```python
from build123d import *

# Parameters (mm, degrees)
SKETCH1_W                = 161
SKETCH1_H                = 100
BOSS_EXTRUDE1_DEPTH      = 12.75
BOSS_EXTRUDE1_DEPTH_BACK = 12.75
SKETCH2_R                = 6.63
SKETCH2_R_2              = 3.525
SKETCH2_R_3              = 1.975
CUT_EXTRUDE1_DEPTH       = 101
FILLET1_R                = 1
FILLET2_R                = 1
FILLET3_R                = 1
FILLET4_R                = 1
SKETCH3_R                = 2.5
BOSS_EXTRUDE2_DEPTH      = 10
SKETCH4_R                = 1.45
CUT_EXTRUDE2_DEPTH       = 5
SKETCH5_W                = 6
SKETCH5_H                = 13
CUT_EXTRUDE3_DEPTH       = 19.25
SKETCH6_R                = 10.25
CUT_EXTRUDE4_DEPTH       = 43.477415469
SKETCH8_R                = 1.5
CUT_EXTRUDE5_DEPTH       = 36.5
SKETCH11_R               = 3
BOSS_EXTRUDE4_DEPTH      = 5
SKETCH12_R               = 1.5
CUT_EXTRUDE7_DEPTH       = 5
SKETCH13_W               = 18.25
SKETCH13_H               = 6
BOSS_EXTRUDE5_DEPTH      = 100
SKETCH14_W               = 4
SKETCH14_H               = 2
BOSS_EXTRUDE6_DEPTH      = 25
BOSS_EXTRUDE6_DEPTH_BACK = 125


with BuildPart() as part:
    # Sketch1 → Boss-Extrude1 (new body, two sides)
    with BuildSketch(Plane(origin=(0, 0, 0), x_dir=(1, 0, 0), z_dir=(0, 1, 0))) as boss_extrude1_sk:
        Rectangle(SKETCH1_W, SKETCH1_H)
    extrude(amount=BOSS_EXTRUDE1_DEPTH)
    extrude(boss_extrude1_sk.sketch, amount=-BOSS_EXTRUDE1_DEPTH_BACK)

    # Sketch2 → Cut-Extrude1 (cut, through all)
    with BuildSketch(Plane.XY.offset(50)):
        with Locations((-67.75, 0)):
            Circle(SKETCH2_R)
        with Locations((67.75, 0)):
            Circle(SKETCH2_R_2)
        with Locations((-75.45, 8.2)):
            Circle(SKETCH2_R_3)
        with Locations((-75.45, -8.2)):
            Circle(SKETCH2_R_3)
        with Locations((-60.05, -8.2)):
            Circle(SKETCH2_R_3)
        with Locations((-60.05, 8.2)):
            Circle(SKETCH2_R_3)
    extrude(amount=-CUT_EXTRUDE1_DEPTH, mode=Mode.SUBTRACT)

    # Fillet1
    fillet1_edges = [part.edges().sort_by_distance(p)[0] for p in [
        (-74.38, 0, -50),
    ]]
    fillet(fillet1_edges, radius=FILLET1_R)

    # Fillet2
    fillet2_edges = [part.edges().sort_by_distance(p)[0] for p in [
        (-74.38, 0, 50),
    ]]
    fillet(fillet2_edges, radius=FILLET2_R)

    # Fillet3
    fillet3_edges = [part.edges().sort_by_distance(p)[0] for p in [
        (64.225, 0, 50),
    ]]
    fillet(fillet3_edges, radius=FILLET3_R)

    # Fillet4
    fillet4_edges = [part.edges().sort_by_distance(p)[0] for p in [
        (64.225, 0, -50),
    ]]
    fillet(fillet4_edges, radius=FILLET4_R)

    # Sketch3 → Boss-Extrude2 (add)
    with BuildSketch(Plane(origin=(0, 12.75, 0), x_dir=(1, 0, 0), z_dir=(0, 1, 0))):
        with Locations((-16.76, 42.46)):
            Circle(SKETCH3_R)
        with Locations((58.37, 42.46)):
            Circle(SKETCH3_R)
        with Locations((-17, -5.8)):
            Circle(SKETCH3_R)
        with Locations((34.7, -0.9)):
            Circle(SKETCH3_R)
        with Locations((65.72, -5.8)):
            Circle(SKETCH3_R)
    extrude(amount=BOSS_EXTRUDE2_DEPTH)

    # Sketch4 → Cut-Extrude2 (cut)
    with BuildSketch(Plane(origin=(0, 22.75, 0), x_dir=(1, 0, 0), z_dir=(0, 1, 0))):
        with Locations((-16.76, 42.46)):
            Circle(SKETCH4_R)
        with Locations((-17, -5.8)):
            Circle(SKETCH4_R)
        with Locations((34.7, -0.9)):
            Circle(SKETCH4_R)
        with Locations((65.72, -5.8)):
            Circle(SKETCH4_R)
        with Locations((58.37, 42.46)):
            Circle(SKETCH4_R)
    extrude(amount=-CUT_EXTRUDE2_DEPTH, mode=Mode.SUBTRACT)

    # Sketch5 → Cut-Extrude3 (cut)
    with BuildSketch(Plane(origin=(80.5, 0, 0), x_dir=(0, 0, -1), z_dir=(1, 0, 0))):
        with Locations((-30, 0)):
            Rectangle(SKETCH5_W, SKETCH5_H)
        with Locations((-10, 0)):
            Rectangle(SKETCH5_W, SKETCH5_H)
        with Locations((10, 0)):
            Rectangle(SKETCH5_W, SKETCH5_H)
        with Locations((30, 0)):
            Rectangle(SKETCH5_W, SKETCH5_H)
    extrude(amount=-CUT_EXTRUDE3_DEPTH, mode=Mode.SUBTRACT)

    # Sketch6 → Cut-Extrude4 (cut, through all)
    with BuildSketch(Plane(origin=(0, 20.916044041, 3.688062894), x_dir=(1, 0, 0), z_dir=(0, 0.984807753, 0.173648178))):
        with Locations((0, -21.249093385)):
            Circle(SKETCH6_R)
    extrude(amount=-CUT_EXTRUDE4_DEPTH, mode=Mode.SUBTRACT)

    # Sketch8 → Cut-Extrude5 (cut, through all)
    with BuildSketch(Plane.XZ.offset(12.75)):
        with Locations((28.5, 2.93086019)):
            Circle(SKETCH8_R)
        with Locations((28.5, 45.38111272)):
            Circle(SKETCH8_R)
        with Locations((-28.5, 2.93086019)):
            Circle(SKETCH8_R)
        with Locations((-28.5, 45.38111272)):
            Circle(SKETCH8_R)
    extrude(amount=-CUT_EXTRUDE5_DEPTH, mode=Mode.SUBTRACT)

    # Sketch11 → Boss-Extrude4 (add)
    with BuildSketch(Plane(origin=(0, 12.75, 0), x_dir=(1, 0, 0), z_dir=(0, 1, 0))):
        with Locations((-38, -6.5)):
            Circle(SKETCH11_R)
        with Locations((-38, -44)):
            Circle(SKETCH11_R)
        with Locations((-75.5, -6.5)):
            Circle(SKETCH11_R)
        with Locations((-75.5, -44)):
            Circle(SKETCH11_R)
    extrude(amount=BOSS_EXTRUDE4_DEPTH)

    # Sketch12 → Cut-Extrude7 (cut)
    with BuildSketch(Plane(origin=(0, 17.75, 0), x_dir=(1, 0, 0), z_dir=(0, 1, 0))):
        with Locations((-75.5, -44)):
            Circle(SKETCH12_R)
        with Locations((-75.5, -6.5)):
            Circle(SKETCH12_R)
        with Locations((-38, -6.5)):
            Circle(SKETCH12_R)
        with Locations((-38, -44)):
            Circle(SKETCH12_R)
    extrude(amount=-CUT_EXTRUDE7_DEPTH, mode=Mode.SUBTRACT)

    # Sketch13 → Boss-Extrude5 (add)
    with BuildSketch(Plane.XY.offset(50)):
        with Locations((89.625, 9.75)):
            Rectangle(SKETCH13_W, SKETCH13_H)
    extrude(amount=-BOSS_EXTRUDE5_DEPTH)

    # Sketch14 → Boss-Extrude6 (add, two sides)
    with BuildSketch(Plane.XY.offset(50)) as boss_extrude6_sk:
        with Locations((100.75, 11.75)):
            Rectangle(SKETCH14_W, SKETCH14_H)
    extrude(amount=BOSS_EXTRUDE6_DEPTH)
    extrude(boss_extrude6_sk.sketch, amount=-BOSS_EXTRUDE6_DEPTH_BACK)


solid = part.part
```
Input: part model. Units: mm. Frame: model coordinates. A direction names the side the tool comes from. Round coordinates to 2 decimals unless told otherwise and drop trailing zeros. Write each loop counter-clockwise with the first axis right and the second up, starting at its lowest first coordinate (ties: lowest second). Pieces come first, ordered by that corner, then holes. Notation, with made-up numbers: (44.5, -21.5) - (66.5, -21.5) arc R24 cw to (66.5, -5.5) - close; hole circle Ø6 at (6.5, 42). An arc over 180 degrees is marked (long way). Write item = value, one per line.
(1) Section query D-D on x = -2. Output: boundary loops of the cut face in (y, z).
Geometry check:
outline = (-12.75, -50) - (12.75, -50) - (12.75, 13.62) - (-12.75, 9.12) - close; (-12.75, 29.54) - (12.75, 34.03) - (12.75, 50) - (-12.75, 50) - close
(2) Section query B-B on z = 39. Output: boundary loops of the cut face in (x, y) (3 decimals).
Geometry check:
outline = (-80.5, -12.75) - (80.5, -12.75) - (80.5, 6.75) - (98.75, 6.75) - (98.75, 10.75) - (102.75, 10.75) - (102.75, 12.75) - (-80.5, 12.75) - close; hole circle Ø3.95 at (-75.45, -8.2); hole circle Ø3.95 at (-75.45, 8.2); hole circle Ø13.26 at (-67.75, 0); hole circle Ø3.95 at (-60.05, -8.2); hole circle Ø3.95 at (-60.05, 8.2); hole circle Ø7.05 at (67.75, 0)
(3) Contact query for flat-ended pins moving along their axis: pin 1 Ø4 at (x, z) = (-38, 44) entering from +Y; pin 2 Ø15 at (x, y) = (-67.75, 0) entering from +Z; pin 3 Ø2.5 at (x, z) = (-75.5, 6.5) entering from +Y. Output: stop coordinate, or through.
Geometry check:
pin_1 = 17.75
pin_2 = 49.99
pin_3 = 12.75
(4) Section query C-C on y = 0. State how many separate pieces and enclosed holes the cut face has, then the cut area to 3 significant figures.
Geometry check:
separate_pieces = 7
enclosed_holes = 5
area = 13,400 mm^2
(5) Material intervals for probe 1 along X at (y, z) = (15, 44); probe 2 along Y at (x, z) = (-60.05, 24) (3 decimals); probe 3 along X at (y, z) = (8, 45.5), sorted ascending.
Geometry check:
probe_1 = -78.5 to -77, -74 to -72.5, -41 to -39.5, -36.5 to -35
probe_2 = -12.75 to -10.175, -6.225 to 6.225, 10.175 to 12.75
probe_3 = -80.5 to -77.41, -73.49 to -62.01, -58.09 to -30, -27 to 27, 30 to 98.75
(6) Access query for faces 1 (the flat face through (61.25, 0, 30)), 2 (the flat face through (101, 10.75, 1)), 3 (the flat face through (58.3, 22.75, -40.8)), 4 (the cylindrical face through (71.1, 1.1, 20.1)), 5 (the cylindrical face through (32.2, 17.7, 0.8)). Directions: +Z, -Z, +X, -X, +Y, -Y. A direction counts if a zero-diameter tool reaches every point of the face in a straight line with its end or side. Return the directions, or none.
Geometry check:
face_1 = +X
face_2 = +Z, -Z, +X, -Y
face_3 = +Z, -Z, +X, -X, +Y
face_4 = +Z, -Z
face_5 = +Y
(7) Pull-direction query (X, two-part tool) for faces 6 (the flat face through (73, 0, 27)), 7 (the cylindrical face through (-73.011, -4.034, 0.686)), 8 (the flat face through (98.75, 9, 1)); classes: +X half, -X half, draft (parallel to the pull), parting line (faces both ways), or undercut.
Geometry check:
face_6 = draft
face_7 = undercut
face_8 = +X half
(8) Section query A-A on x = -67.75. Output: boundary loops of the cut face in (y, z), then the cut area to 3 significant figures.
Geometry check:
outline = (-12.75, -50) - (-7.63, -50) arc R1 ccw to (-6.63, -49) - (-6.63, 49) arc R1 ccw to (-7.63, 50) - (-12.75, 50) - close; (6.63, -49) arc R1 ccw to (7.63, -50) - (12.75, -50) - (12.75, 50) - (7.63, 50) arc R1 ccw to (6.63, 49) - close
area = 1,220 mm^2
